Source: CAD feature listing. Evaluate the final solid. Frame: model axes, mm. Face numbers are marked on the shaded views. A direction names the side the tool comes from. Round coordinates to 2 decimals unless told otherwise and drop trailing zeros. Order: outer loops, then holes, each group sorted by start corner. A loop starts at its lowest first (then second) coordinate and runs counter-clockwise, first axis right, second up. Notation, with made-up numbers: M 37,-39 L 90,-39 A21 ccw 90,-33 Z; hole C 53,9.5 d4. An arc over 180 degrees is marked long. Use one line per item in the form item = value. Start each with the question number.
Q1. Reachability of the marked faces 3 and 4 from +Z, -Z, +X, -X, +Y, -Y: full face, straight path, thin tool, end or side. Return the list, or none.
Q2. Material intervals for probe 1 along Y at (x, z) = (0, 4.25); probe 2 along Y at (x, z) = (0, 382); probe 3 along Z at (x, y) = (-89, -72), sorted ascending.
Q3. Section A-A (z = 70). Return the cut outline in (x, y), plus the area to 3 significant figures.
Q4. Pull-direction query (X, two-part tool) for the marked faces 1 and 2; classes: pulls with the +X half, pulls with the -X half, needs draft (parallel to the pull), parting line crosses it, or undercut.
Q5. Section B-B (y = -67). Give the number of separate pieces and of enclosed holes in the cut face, plus the area to 3 significant figures.
Q6. Section C-C (z = 351). Return the cut outline in (x, y).
Q7. Contact query for flat-ended pins moving along their axis: pin 1 (1.5 mm diameter, centred on x = 14, z = 72.5, fed in from -Y); pin 2 (5 mm diameter, centred on y = -69, z = 329, fed in from -X). Output: stop coordinate, or through.
from build123d import *

# Parameters (mm, degrees)
SKETCH1_R       = 119.4
SKETCH1_R_2     = 117.4
EXTRUDE1_DEPTH  = 10
SKETCH2_R       = 119.4
SKETCH2_R_2     = 118.4
EXTRUDE2_DEPTH  = 5
SKETCH3_R       = 119.4
SKETCH3_R_2     = 117.4
EXTRUDE3_DEPTH  = 15
SKETCH4_R       = 118.4
SKETCH4_R_2     = 117.4
EXTRUDE4_DEPTH  = 10
EXTRUDE5_DEPTH  = 240
SKETCH6_R       = 118.4
SKETCH6_R_2     = 117.4
EXTRUDE6_DEPTH  = 30
SKETCH7_R       = 118.4
SKETCH7_R_2     = 109.4
EXTRUDE7_DEPTH  = 2
SKETCH8_R       = 111.4
SKETCH8_R_2     = 109.4
EXTRUDE8_DEPTH  = 60
SKETCH9_R       = 111.4
SKETCH9_R_2     = 102.5
EXTRUDE9_DEPTH  = 2
SKETCH10_R      = 104.5
SKETCH10_R_2    = 102.5
EXTRUDE10_DEPTH = 15


with BuildPart() as part:
    # Sketch1 → Extrude1 (new body)
    with BuildSketch(Plane.XY):
        Circle(SKETCH1_R)
        Circle(SKETCH1_R_2, mode=Mode.SUBTRACT)
    extrude(amount=EXTRUDE1_DEPTH)

    # Sketch2 → Extrude2 (add)
    with BuildSketch(Plane.XY.offset(10)):
        Circle(SKETCH2_R)
        Circle(SKETCH2_R_2, mode=Mode.SUBTRACT)
    extrude(amount=EXTRUDE2_DEPTH)

    # Sketch3 → Extrude3 (add)
    with BuildSketch(Plane.XY.offset(15)):
        Circle(SKETCH3_R)
        Circle(SKETCH3_R_2, mode=Mode.SUBTRACT)
    extrude(amount=EXTRUDE3_DEPTH)

    # Sketch4 → Extrude4 (add)
    with BuildSketch(Plane.XY.offset(30)):
        Circle(SKETCH4_R)
        Circle(SKETCH4_R_2, mode=Mode.SUBTRACT)
    extrude(amount=EXTRUDE4_DEPTH)

    # Sketch5 → Extrude5 (add)
    with BuildSketch(Plane.XY.offset(40)):
        with BuildLine():
            Line((20.559944, 116.601238), (20.386296, 115.61643))
            ThreePointArc((20.386296, 115.61643), (0, 117.4), (-20.386296, 115.61643))
            Line((-20.386296, 115.61643), (-20.559944, 116.601238))
            ThreePointArc((-20.559944, 116.601238), (0, 118.4), (20.559944, 116.601238))
        make_face()
        with BuildLine():
            Line((116.601238, 20.559944), (115.61643, 20.386296))
            ThreePointArc((115.61643, 20.386296), (117.4, 0), (115.61643, -20.386296))
            Line((115.61643, -20.386296), (116.601238, -20.559944))
            ThreePointArc((116.601238, -20.559944), (118.4, 0), (116.601238, 20.559944))
        make_face()
        with BuildLine():
            Line((20.559944, -116.601238), (20.386296, -115.61643))
            ThreePointArc((20.386296, -115.61643), (0, -117.4), (-20.386296, -115.61643))
            Line((-20.386296, -115.61643), (-20.559944, -116.601238))
            ThreePointArc((-20.559944, -116.601238), (0, -118.4), (20.559944, -116.601238))
        make_face()
        with BuildLine():
            Line((-115.61643, -20.386296), (-116.601238, -20.559944))
            ThreePointArc((-116.601238, -20.559944), (-118.4, 0), (-116.601238, 20.559944))
            Line((-116.601238, 20.559944), (-115.61643, 20.386296))
            ThreePointArc((-115.61643, 20.386296), (-117.4, 0), (-115.61643, -20.386296))
        make_face()
    extrude(amount=EXTRUDE5_DEPTH)

    # Sketch6 → Extrude6 (add)
    with BuildSketch(Plane.XY.offset(280)):
        Circle(SKETCH6_R)
        Circle(SKETCH6_R_2, mode=Mode.SUBTRACT)
    extrude(amount=EXTRUDE6_DEPTH)

    # Sketch7 → Extrude7 (add)
    with BuildSketch(Plane.XY.offset(310)):
        Circle(SKETCH7_R)
        Circle(SKETCH7_R_2, mode=Mode.SUBTRACT)
    extrude(amount=EXTRUDE7_DEPTH)

    # Sketch8 → Extrude8 (add)
    with BuildSketch(Plane.XY.offset(312)):
        Circle(SKETCH8_R)
        Circle(SKETCH8_R_2, mode=Mode.SUBTRACT)
    extrude(amount=EXTRUDE8_DEPTH)

    # Sketch9 → Extrude9 (add)
    with BuildSketch(Plane.XY.offset(372)):
        Circle(SKETCH9_R)
        Circle(SKETCH9_R_2, mode=Mode.SUBTRACT)
    extrude(amount=-EXTRUDE9_DEPTH)

    # Sketch10 → Extrude10 (add)
    with BuildSketch(Plane.XY.offset(372)):
        Circle(SKETCH10_R)
        Circle(SKETCH10_R_2, mode=Mode.SUBTRACT)
    extrude(amount=EXTRUDE10_DEPTH)


solid = part.part
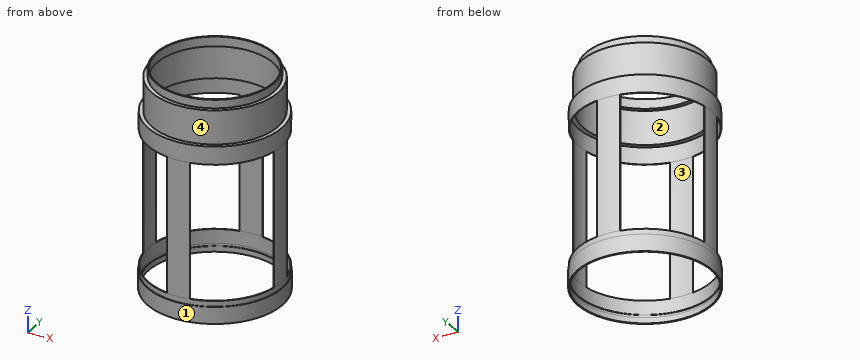
Results list:
q1.face_3 = -Z
q1.face_4 = +Z
q2.probe_1 = -119.4 to -117.4, 117.4 to 119.4
q2.probe_2 = -104.5 to -102.5, 102.5 to 104.5
q2.probe_3 = 310 to 312
q3.outline = M -116.6,-20.56 L -115.62,-20.39 A117.4 cw -115.62,20.39 L -116.6,20.56 A118.4 ccw Z; M -20.56,-116.6 A118.4 ccw 20.56,-116.6 L 20.39,-115.62 A117.4 cw -20.39,-115.62 Z; M -20.56,116.6 L -20.39,115.62 A117.4 cw 20.39,115.62 L 20.56,116.6 A118.4 ccw Z; M 115.62,-20.39 L 116.6,-20.56 A118.4 ccw 116.6,20.56 L 115.62,20.39 A117.4 cw Z
q3.area = 165 mm2
q4.face_1 = parting line crosses it
q4.face_2 = undercut
q5.separate_pieces = 4
q5.enclosed_holes = 0
q5.area = 692 mm2
q6.outline = C 0,0 d222.8; hole C 0,0 d218.8
q7.pin_1 = -117.66
q7.pin_2 = -89.37
